For this review, take the finished solid that the model builds, in its own axes (mm). Face numbers are marked on the shaded views. A direction names the side the tool comes from. Give positions to 0.01 mm unless a question says otherwise; leave off trailing zeros. Write each loop counter-clockwise with the first axis right and the second up, starting at its lowest first coordinate (ties: lowest second). Pieces come first, ordered by that corner, then holes. Notation, with made-up numbers: (-6, -22.5) -> (24, -22.5) arc R16 cw to (24, -17.5) -> close; hole circle Ø7 at (-11, -6). An arc over 180 degrees is marked (long way). Return JSON: item names as keys, results as strings.
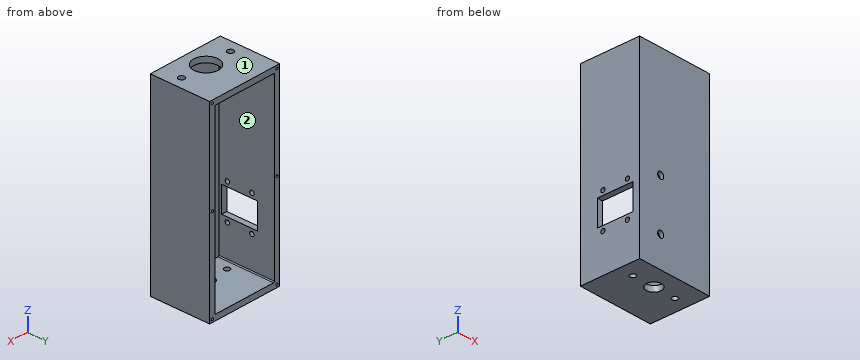
from build123d import *

# Parameters (mm, degrees)
SKETCH_1_W             = 80
SKETCH_1_H             = 48
EXTRUDE_1_DEPTH        = 200
CUT_EXTRUDE_1_DEPTH    = 44
SKETCH_3_R             = 3.3
SKETCH_3_R_2           = 13
CUT_EXTRUDE_2_DEPTH    = 10
SKETCH_4_R             = 2.25
SKETCH_4_W             = 27
SKETCH_4_H             = 38
CUT_EXTRUDE_3_DEPTH    = 10
SKETCH_5_R             = 8
SKETCH_5_R_2           = 3
CUT_EXTRUDE_4_DEPTH    = 10
SKETCH_6_R             = 3.500000002
SKETCH_6_R_2           = 3.5
CUT_EXTRUDE_5_DEPTH    = 10
SKETCH_8_W             = 80
SKETCH_8_H             = 200
EXTRUDE_2_DEPTH        = 15
HOLE_WIZARD_M3_1_D     = 2.5
HOLE_WIZARD_M3_1_DEPTH = 7.5
HOLE_WIZARD_M3_1_TIP   = 0.751075774


with BuildPart() as part:
    # 草图1 → 凸台-拉伸1 (new body)
    with BuildSketch(Plane.XY):
        Rectangle(SKETCH_1_W, SKETCH_1_H)
    extrude(amount=-EXTRUDE_1_DEPTH)

    # 草图2 → 切除-拉伸1 (cut)
    with BuildSketch(Plane(origin=(0, 24, 0), x_dir=(1, 0, 0), z_dir=(0, 1, 0))):
        with BuildLine():
            ThreePointArc((-34, 193), (-33.707106781, 193.707106781), (-33, 194))
            Line((-33, 194), (33, 194))
            ThreePointArc((33, 194), (33.707106781, 193.707106781), (34, 193))
            Line((34, 193), (34, 7))
            ThreePointArc((34, 7), (33.707106781, 6.292893219), (33, 6))
            Line((33, 6), (-33, 6))
            ThreePointArc((-33, 6), (-33.707106781, 6.292893219), (-34, 7))
            Line((-34, 7), (-34, 193))
        make_face()
    extrude(amount=-CUT_EXTRUDE_1_DEPTH, mode=Mode.SUBTRACT)

    # 草图3 → 切除-拉伸2 (cut)
    with BuildSketch(Plane.XY):
        with Locations((-28, -2)):
            Circle(SKETCH_3_R)
        with Locations((0, -2)):
            Circle(SKETCH_3_R_2)
        with Locations((28, -2)):
            Circle(SKETCH_3_R)
    extrude(amount=-CUT_EXTRUDE_2_DEPTH, mode=Mode.SUBTRACT)

    # 草图4 → 切除-拉伸3 (cut)
    with BuildSketch(Plane.ZY.offset(40)):
        with Locations((-123, -11)):
            Circle(SKETCH_4_R)
        with Locations((-123, 15)):
            Circle(SKETCH_4_R)
        with Locations((-160, 15)):
            Circle(SKETCH_4_R)
        with Locations((-160, -11)):
            Circle(SKETCH_4_R)
        with Locations((-141.5, 2)):
            Rectangle(SKETCH_4_W, SKETCH_4_H)
    extrude(amount=-CUT_EXTRUDE_3_DEPTH, mode=Mode.SUBTRACT)

    # 草图5 → 切除-拉伸4 (cut)
    with BuildSketch(Plane(origin=(0, 0, -200), x_dir=(-1, 0, 0), z_dir=(0, 0, -1))):
        with Locations((0, -2)):
            Circle(SKETCH_5_R)
        with Locations((24, -2)):
            Circle(SKETCH_5_R_2)
        with Locations((-24, -2)):
            Circle(SKETCH_5_R_2)
    extrude(amount=-CUT_EXTRUDE_4_DEPTH, mode=Mode.SUBTRACT)

    # 草图6 → 切除-拉伸5 (cut)
    with BuildSketch(Plane(origin=(0, -20, 0), x_dir=(1, 0, 0), z_dir=(0, 1, 0))):
        with Locations((-16, 168)):
            Circle(SKETCH_6_R)
        with Locations((-16, 115)):
            Circle(SKETCH_6_R_2)
    extrude(amount=-CUT_EXTRUDE_5_DEPTH, mode=Mode.SUBTRACT)

    # 草图8 → 凸台-拉伸2 (add)
    with BuildSketch(Plane(origin=(0, 24, 0), x_dir=(1, 0, 0), z_dir=(0, 1, 0))):
        with Locations((0, 100)):
            Rectangle(SKETCH_8_W, SKETCH_8_H)
        with BuildLine():
            Line((-33, 6), (33, 6))
            ThreePointArc((33, 6), (33.707106781, 6.292893219), (34, 7))
            Line((34, 7), (34, 193))
            ThreePointArc((34, 193), (33.707106781, 193.707106781), (33, 194))
            Line((33, 194), (-33, 194))
            ThreePointArc((-33, 194), (-33.707106781, 193.707106781), (-34, 193))
            Line((-34, 193), (-34, 7))
            ThreePointArc((-34, 7), (-33.707106781, 6.292893219), (-33, 6))
        make_face(mode=Mode.SUBTRACT)
    extrude(amount=EXTRUDE_2_DEPTH)

    # M3 螺纹孔1
    with Locations(Plane(origin=(-37, 39, -100), x_dir=(0, 0, 1), z_dir=(0, 1, 0))):
        with Locations((0, 0), (0, 74), (97, 74), (97, 0), (-97, 0), (-97, 74)):
            Hole(HOLE_WIZARD_M3_1_D / 2, depth=HOLE_WIZARD_M3_1_DEPTH)
            with Locations((0, 0, -(HOLE_WIZARD_M3_1_DEPTH + HOLE_WIZARD_M3_1_TIP / 2))):  # 118° drill point
                Cone(0, HOLE_WIZARD_M3_1_D / 2, HOLE_WIZARD_M3_1_TIP, mode=Mode.SUBTRACT)


solid = part.part
1. For the marked faces 1 and 2, list the 3-axis set-ups (+Z, -Z, +X, -X, +Y, -Y) from which the entire face can be reached by the end or side of a thin tool; tool diameter is ignored.
Results found:
{"face 1": "+Z, +X, -X, +Y, -Y", "face 2": "+Y"}
2. Add section D-D, the plane x = 2. State the section outline as (y, z) points.
Results found:
{"outline": "(-24, -200) -> (-9.75, -200) -> (-9.75, -194) -> (-20, -194) -> (-20, -6) -> (-14.85, -6) -> (-14.85, 0) -> (-24, 0) -> close; (5.75, -200) -> (39, -200) -> (39, -194) -> (5.75, -194) -> close; (10.85, -6) -> (39, -6) -> (39, 0) -> (10.85, 0) -> close"}
3. To check wall thickness, follow probe 1 along Z at (x, y) = (37, 37.25); probe 2 along Y at (x, z) = (-35.5, -160); probe 3 along X at (y, z) = (35, -3). State the ranges of each line that lie inside material, in increasing order.
Results found:
{"probe 1": "z = -200 to -198.25, -195.75 to -101.25, -98.75 to -4.25, -1.75 to 0", "probe 2": "y = -24 to -13.25, -8.75 to 12.75, 17.25 to 39", "probe 3": "x = -40 to -38.25, -35.75 to 35.75, 38.25 to 40"}
4. Add section C-C, the plane z = -26.5. State the section outline as (x, y) points, plus the area to 3 significant figures.
Results found:
{"outline": "(-40, -24) -> (40, -24) -> (40, 39) -> (34, 39) -> (34, -20) -> (-34, -20) -> (-34, 39) -> (-40, 39) -> close", "area": "1,030 mm²"}
5. For pin 1 (2 mm diameter, centred on x = -37, z = -3, fed in from +Y); pin 2 (9 mm diameter, centred on x = -16, z = -168, fed in from +Y); pin 3 (10.5 mm diameter, centred on x = -28, y = -2, fed in from +Z); pin 4 (4 mm diameter, centred on y = -11, z = -160, fed in from -X), all flat-tipped, find the tip position at first contact; note any pin that passes through.
Results found:
{"pin 1": "stops at y = 31.35", "pin 2": "stops at y = -20", "pin 3": "stops at z = 0", "pin 4": "stops at x = 34"}
6. Add section B-B, the plane y = 15. State the section outline as (x, z) points.
Results found:
{"outline": "(-40, -200) -> (40, -200) -> (40, 0) -> (-40, 0) -> (-40, -120.75) -> (-34, -120.75) -> (-34, -7) arc R1 cw to (-33, -6) -> (33, -6) arc R1 cw to (34, -7) -> (34, -193) arc R1 cw to (33, -194) -> (-33, -194) arc R1 cw to (-34, -193) -> (-34, -162.25) -> (-40, -162.25) -> close; (-40, -157.75) -> (-34, -157.75) -> (-34, -155) -> (-40, -155) -> close; (-40, -128) -> (-34, -128) -> (-34, -125.25) -> (-40, -125.25) -> close"}
7. Add section A-A, the plane z = -152. State the section outline as (x, y) points, plus the area to 3 significant figures.
Results found:
{"outline": "(-40, -24) -> (40, -24) -> (40, 39) -> (34, 39) -> (34, -20) -> (-34, -20) -> (-34, -17) -> (-40, -17) -> close; (-40, 21) -> (-34, 21) -> (-34, 39) -> (-40, 39) -> close", "area": "800 mm²"}
